Autodesk Inventor part; units mm, degrees
ref_plane "YZ Plane" through (0, 0, 0) normal (1, 0, 0) x (0, 1, 0)
ref_plane "XZ Plane" through (0, 0, 0) normal (0, 1, 0) x (-1, 0, 0)
ref_plane "XY Plane" through (0, 0, 0) normal (0, 0, 1) x (1, 0, 0)
sketch "Эскиз1" plane through (0, 0, 0) normal (0, 0, 1) x (1, 0, 0)
  line L0 (0, 0) -> (35, 0)
  line L1 (35, 0) -> (35, 20)
  line L2 (35, 20) -> (0, 20)
  line L3 (0, 20) -> (0, 0)
  dimension "d0" = 35
  dimension "d1" = 20
extrude "Выдавливание1" add sketch "Эскиз1" along normal blind 1.5
sketch "Эскиз2" plane through (0, 0, 1.5) normal (0, 0, 1) x (1, 0, 0)
  line L0 (0, 20) -> (0, 0)
  line L1 (0, 0) -> (5, 0)
  line L2 (5, 0) -> (5, 5)
  line L3 (5, 5) -> (0, 5)
  line L4 (0, 5) -> (0, 0)
  line L5 (35, 20) -> (0, 20)
  line L6 (0, 20) -> (5, 20)
  line L7 (5, 20) -> (5, 15)
  line L8 (5, 15) -> (0, 15)
  line L9 (0, 15) -> (0, 20)
  dimension "d4" = 5
  dimension "d5" = 5
  dimension "d6" = 5
  dimension "d7" = 5
extrude "Выдавливание2" add sketch "Эскиз2" along normal blind 6
sketch "Эскиз3" plane through (0, 0, 7.5) normal (0, 0, 1) x (1, 0, 0)
  circle A0 centre (1.8, 1.8) radius 0.75
  circle A1 centre (1.8, 18.2) radius 0.75
  line L0 (0, 0) -> (5, 0)
  line L1 (0, 5) -> (0, 0)
  line L2 (0, 20) -> (0, 15)
  line L3 (5, 20) -> (0, 20)
  dimension "d10" = 1.5
  dimension "d11" = 1.5
  dimension "d12" = 1.8
  dimension "d13" = 1.8
  dimension "d14" = 1.8
  dimension "d15" = 1.8
extrude "Выдавливание3" cut sketch "Эскиз3" against normal blind 6
fillet "Сопряжение1" radius 2 4 edges at (0, 0, 3.75) (0, 20, 3.75) (35, 20, 0.75) (35, 0, 0.75)
properties part number "RDC1-0014_Holder"
Here's how the part is built. I have some questions about the finished solid (model axes, mm). A direction names the side the tool comes from. Give positions to 0.01 mm unless a question says otherwise; leave off trailing zeros. Write each loop counter-clockwise with the first axis right and the second up, starting at its lowest first coordinate (ties: lowest second). Pieces come first, ordered by that corner, then holes. Notation, with made-up numbers: (-20.5, 58.5) -> (-0.5, 58.5) arc R18 cw to (-0.5, 85.5) -> close; hole circle Ø1 at (1.5, 16). An arc over 180 degrees is marked (long way). Use one line per item in the form item = value. Start each with the question number.
1. Imagine slicing it at A-A on z = 2.25. List the corners of the cut face in (x, y) for me.
2. If I drill on L1, parallel to Y at x = 1.8, z = 3.35; L2, parallel to X at y = 3.75, z = 3.5; L3, parallel to Z at x = 11, y = 17.75, over which ranges is the centre line in solid material (lowest first)?
3. Imagine slicing it at C-C on y = 9.75. List the corners of the cut face in (x, z) for me.
4. Thinking about a two-plate mould opening in X: for faces 4 (the face through (2.5, 17.5, 7.5)), 5 (the face through (2, 18, 1.5)), 6 (the face through (5, 18, 4)), which applies, +X half, -X half, draft (parallel to the pull), parting line (faces both ways), or undercut?
5. On a 3-axis mill with a long thin cutter (end or side, diameter ignored), from which of +Z, -Z, +X, -X, +Y, -Y can I reach the whole of each face in a straight line? I mean faces 1 (the face through (3, 15, 4)), 2 (the face through (5, 2, 4)), 3 (the face through (2.146, 1.135, 4.542)). Say none if no direction works.
6. Will these pins go through, and if not, where does the flat tip stop? pin 1 Ø6 at (x, y) = (22.5, 9) entering from +Z; pin 2 Ø4 at (y, z) = (2, 4.5) entering from +X.
7. Imagine slicing it at B-B on x = 7. List the corners of the cut face in (y, z) for me, plus the area to 3 significant figures.
Entries:
q1.outline = (0, 2) arc R2 ccw to (2, 0) -> (5, 0) -> (5, 5) -> (0, 5) -> close; (0, 15) -> (5, 15) -> (5, 20) -> (2, 20) arc R2 ccw to (0, 18) -> close; hole circle Ø1.5 at (1.8, 1.8); hole circle Ø1.5 at (1.8, 18.2)
q2.L1 = 0.01 to 1.05, 2.55 to 5, 15 to 17.45, 18.95 to 19.99
q2.L2 = 0 to 5
q2.L3 = 0 to 1.5
q3.outline = (0, 0) -> (35, 0) -> (35, 1.5) -> (0, 1.5) -> close
q4.face_4 = draft
q4.face_5 = undercut
q4.face_6 = +X half
q5.face_1 = +Z, +X, -X
q5.face_2 = +Z, +X, +Y, -Y
q5.face_3 = +Z
q6.pin_1 = 1.5
q6.pin_2 = 5
q7.outline = (0, 0) -> (20, 0) -> (20, 1.5) -> (0, 1.5) -> close
q7.area = 30.0 mm²
